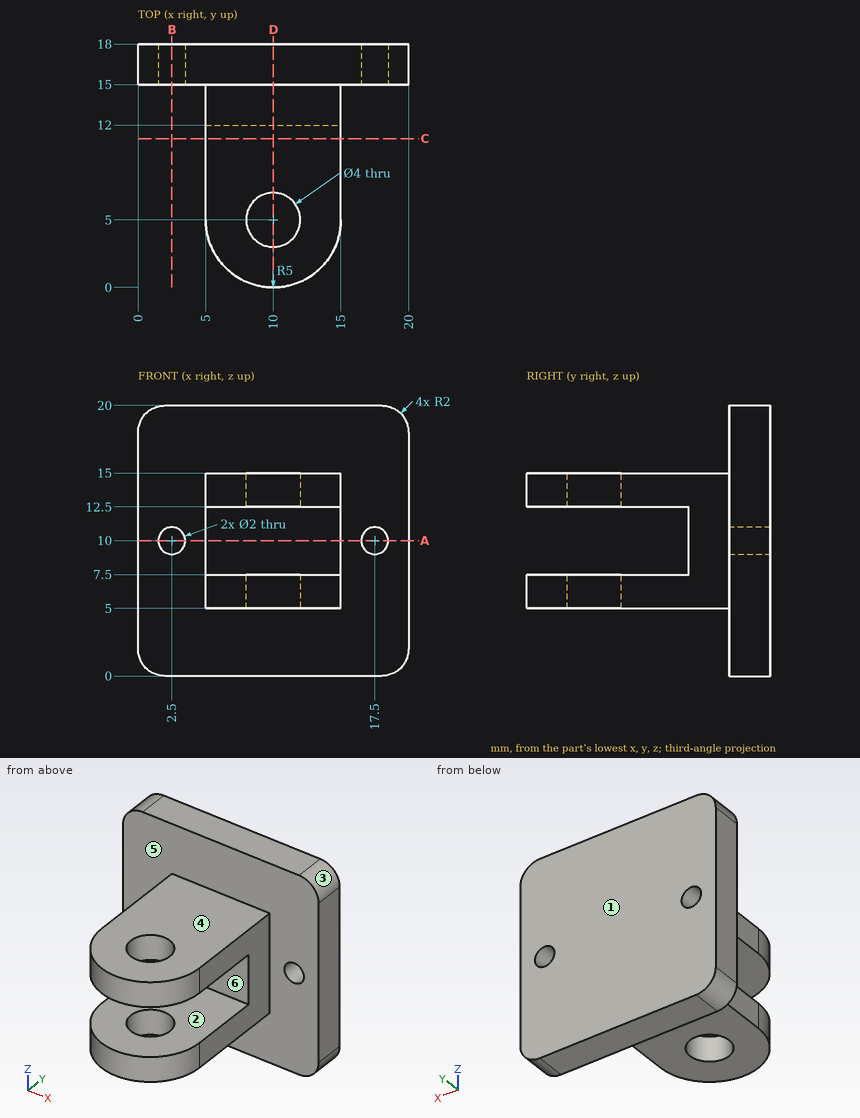
The figure shows three views and two pictorial views of one solid part (mm, origin at its lowest corner). Answer the questions. A direction names the side the tool comes from. Coordinates: 2 decimals unless noted, no trailing zeros. Loops run counter-clockwise (first coordinate to the right, second up) from the corner with the lowest first, then second, coordinate; pieces in that order, holes last.
1) Find section D-D on x = 10. Write down the section's boundary in (y, z), then the cut area to 3 significant figures.
2) Find section C-C on y = 11. Write down the section's boundary in (x, z).
3) A tool of negligible diameter and unlimited length cuts with its end or side. For the marked faces 4, 5 and 6, from which of +Z, -Z, +X, -X, +Y, -Y can it reach the whole face along a straight path? Write none if from no direction.
4) Find the intervals of material crossed by L1, parallel to X at y = 16.95, z = 10; L2, parallel to Y at x = 10, z = 5.8; L3, parallel to X at y = 8.25, z = 6.5, in increasing order.
5) Find section B-B on x = 2.5. Write down the section's boundary in (y, z), then the cut area to 3 significant figures.
6) Flat-ended cylindrical pins translate along their axes: pin 1 Ø6 at (x, z) = (3.5, 2) entering from -Y; pin 2 Ø1.8 at (x, z) = (17.5, 10) entering from +Y; pin 3 Ø5 at (x, y) = (8.5, 8.5) entering from -Z; pin 4 Ø3 at (x, y) = (11, 9) entering from +Z. Find the tip coordinate at first contact, or state that the pin passes through.
7) Determine the mould class of the marked faces 1, 2 and 3 for opening direction Z: pulls with the +Z half, pulls with the -Z half, needs draft (parallel to the pull), parting line crosses it, or undercut.
8) Find section A-A on z = 10. Write down the section's boundary in (x, y).
Values:
1. outline: (0, 5) - (3, 5) - (3, 7.5) - (0, 7.5) - close; (0, 12.5) - (3, 12.5) - (3, 15) - (0, 15) - close; (7, 5) - (15, 5) - (15, 0) - (18, 0) - (18, 20) - (15, 20) - (15, 15) - (7, 15) - (7, 12.5) - (12, 12.5) - (12, 7.5) - (7, 7.5) - close
1. area: 130 mm2
2. outline: (5, 5) - (15, 5) - (15, 7.5) - (5, 7.5) - close; (5, 12.5) - (15, 12.5) - (15, 15) - (5, 15) - close
3. face 4: +Z, +X, -X, -Y
3. face 5: -Y
3. face 6: +X, -X, -Y
4. L1: x = 0 to 1.5, 3.5 to 16.5, 18.5 to 20
4. L2: y = 0 to 3, 7 to 18
4. L3: x = 5 to 15
5. outline: (15, 0) - (18, 0) - (18, 9) - (15, 9) - close; (15, 11) - (18, 11) - (18, 20) - (15, 20) - close
5. area: 54.0 mm2
6. pin 1: stops at y = 15
6. pin 2: passes through
6. pin 3: stops at z = 5
6. pin 4: stops at z = 15
7. face 1: needs draft
7. face 2: undercut
7. face 3: pulls with the +Z half
8. outline: (0, 15) - (1.5, 15) - (1.5, 18) - (0, 18) - close; (3.5, 15) - (5, 15) - (5, 12) - (15, 12) - (15, 15) - (16.5, 15) - (16.5, 18) - (3.5, 18) - close; (18.5, 15) - (20, 15) - (20, 18) - (18.5, 18) - close
